Geometry check sheet. Reference: the model listing, model coordinates, mm. Face numbers are marked on the shaded views. A direction names the side the tool comes from. Give positions to 0.01 mm unless a question says otherwise; leave off trailing zeros. Write each loop counter-clockwise with the first axis right and the second up, starting at its lowest first coordinate (ties: lowest second). Pieces come first, ordered by that corner, then holes. Notation, with made-up numbers: (3, -3) -> (11, -3) arc R32 cw to (11, 30) -> close; hole circle Ø5 at (54, 43.25). An arc over 180 degrees is marked (long way). Use a Markdown table: item, result. Add a question column.
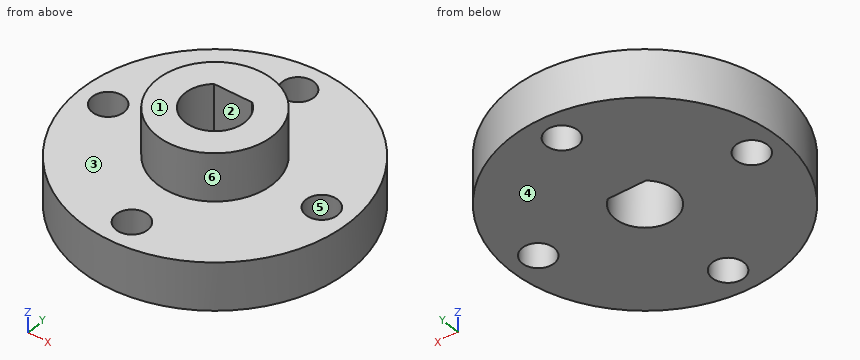
from build123d import *

# Parameters (mm, degrees)
SKETCH1_R           = 14
SKETCH1_R_2         = 1.65
BOSS_EXTRUDE1_DEPTH = 5
SKETCH2_R           = 6
BOSS_EXTRUDE2_DEPTH = 5
CUT_EXTRUDE1_DEPTH  = 11


with BuildPart() as part:
    # Sketch1 → Boss-Extrude1 (new body)
    with BuildSketch(Plane.XY):
        Circle(SKETCH1_R)
        with Locations((0, 11)):
            Circle(SKETCH1_R_2, mode=Mode.SUBTRACT)
        with Locations((11, 0)):
            Circle(SKETCH1_R_2, mode=Mode.SUBTRACT)
        with Locations((0, -11)):
            Circle(SKETCH1_R_2, mode=Mode.SUBTRACT)
        with Locations((-11, 0)):
            Circle(SKETCH1_R_2, mode=Mode.SUBTRACT)
    extrude(amount=BOSS_EXTRUDE1_DEPTH)

    # Sketch2 → Boss-Extrude2 (add)
    with BuildSketch(Plane.XY.offset(5)):
        Circle(SKETCH2_R)
    extrude(amount=BOSS_EXTRUDE2_DEPTH)

    # Sketch3 → Cut-Extrude1 (cut, through all)
    with BuildSketch(Plane.XY.offset(10)):
        with BuildLine():
            Line((-1.962141687, 2.4), (1.962141687, 2.4))
            ThreePointArc((1.962141687, 2.4), (0, -3.1), (-1.962141687, 2.4))
        make_face()
    extrude(amount=-CUT_EXTRUDE1_DEPTH, mode=Mode.SUBTRACT)


solid = part.part
1) Draft check along Y on the marked faces 4, 5 and 6. Enter one of: +Y half, -Y half, draft (parallel to the pull), parting line (faces both ways), or undercut.
2) Sectioned sample at D-D, the plane z = 7.75. Enter the section's corners in (x, y), and give its area (3 significant figures).
3) Gauge pin test, flat ends, axial feed: P1, Ø3, axis at x = 0, y = -11, coming from the -Z side; P2, Ø6, axis at y = -5, z = 8.5, coming from the -X side; P3, Ø6, axis at y = -7, z = 1.5, coming from the -X side; P4, Ø1.5, axis at x = -8, z = 4.5, coming from the +Y side. Record the tip position at first contact, or that the pin passes through.
4) Material ranges on probe 1 along X at (y, z) = (-0.75, 3); probe 2 along Z at (x, y) = (3, 12.5); probe 3 along Y at (x, z) = (11, 3.7), recorded low to high. Write a range as [from, to].
5) Sectioned sample at A-A, the plane x = 11. Enter the section's corners in (y, z).
6) Tool access check on the marked faces 1, 2 and 3. Record the directions out of +Z, -Z, +X, -X, +Y, -Y that give a thin tool (end or side, any length) a straight path to the whole face; none if there is none.
7) Sectioned sample at B-B, the plane x = 0. Enter the section's corners in (y, z), and give its area (3 significant figures).
Check values:
| question | item | result |
|---|---|---|
| 1 | face 4 | draft |
| 1 | face 5 | undercut |
| 1 | face 6 | parting line |
| 2 | outline | circle Ø12 at (0, 0); hole (-1.96, 2.4) arc R3.1 ccw (long way) to (1.96, 2.4) -> close |
| 2 | area | 84.8 mm² |
| 3 | P1 | through |
| 3 | P2 | x = -5.66 |
| 3 | P3 | x = -13.42 |
| 3 | P4 | y = 11.98 |
| 4 | probe 1 | [-13.98, -12.47], [-9.53, -3.01], [3.01, 9.53], [12.47, 13.98] |
| 4 | probe 2 | [0, 5] |
| 4 | probe 3 | [-8.66, -1.65], [1.65, 8.66] |
| 5 | outline | (-8.66, 0) -> (-1.65, 0) -> (-1.65, 5) -> (-8.66, 5) -> close; (1.65, 0) -> (8.66, 0) -> (8.66, 5) -> (1.65, 5) -> close |
| 6 | face 1 | +Z, +X, -X, +Y, -Y |
| 6 | face 2 | +Z, -Z |
| 6 | face 3 | +Z |
| 7 | outline | (-14, 0) -> (-12.65, 0) -> (-12.65, 5) -> (-14, 5) -> close; (-9.35, 0) -> (-3.1, 0) -> (-3.1, 10) -> (-6, 10) -> (-6, 5) -> (-9.35, 5) -> close; (2.4, 0) -> (9.35, 0) -> (9.35, 5) -> (6, 5) -> (6, 10) -> (2.4, 10) -> close; (12.65, 0) -> (14, 0) -> (14, 5) -> (12.65, 5) -> close |
| 7 | area | 112 mm² |
